Check sheet for the modelled part. Datum: model origin and axes. Units: mm. Face numbers are marked on the shaded views. A direction names the side the tool comes from. Coordinates: 2 decimals unless noted, no trailing zeros. Loops run counter-clockwise (first coordinate to the right, second up) from the corner with the lowest first, then second, coordinate; pieces in that order, holes last. Notation, with made-up numbers: (29, 20) -> (52, 20) arc R19 ccw to (52, 31) -> close; hole circle Ø6 at (83, 2.25). An arc over 180 degrees is marked (long way). Use one line per item in the form item = value.
from build123d import *

# Parameters (mm, degrees)
F3_W     = 10.7
F3_H     = 4
F4_DEPTH = 4
F5_R     = 1.99999


# Not quite as in the source:
# - a fillet or chamfer is up to 0.001 mm smaller than in the source, because OpenCascade refuses the exact size


with BuildPart() as f1:
    # F0 (on Front) → F1 (revolve)
    with BuildSketch(Plane.XZ):
        Polygon((0, 8), (0, 0), (215, 0), (215, 5), (203.5, 5), (203.5, 6), (187.5, 6), (187.5, 7.5), (172.5, 7.5), (172.5, 10.75), (168, 10.75), (168, 5.675), (161, 5.675), (161, 8), align=None)
    revolve(axis=Axis((-30.1147408886, 0, 0), (-1, 0, 0)))

    # F3 (on offset) → F4 (cut)
    with BuildSketch(Plane.XY.offset(7.5)):
        with Locations((196.15, 0)):
            Rectangle(F3_W, F3_H)
    extrude(amount=-F4_DEPTH, mode=Mode.SUBTRACT)

    # F5 (radius 2 in the source; OpenCascade refuses exactly that, so slightly less here)
    f5_edges = [f1.edges().sort_by_distance(p)[0] for p in [
        (190.8, 2, 4.578427),
        (201.5, 2, 4.578427),
        (201.5, -2, 4.578427),
        (190.8, -2, 4.578427),
    ]]
    fillet(f5_edges, radius=F5_R)


solid = f1.part
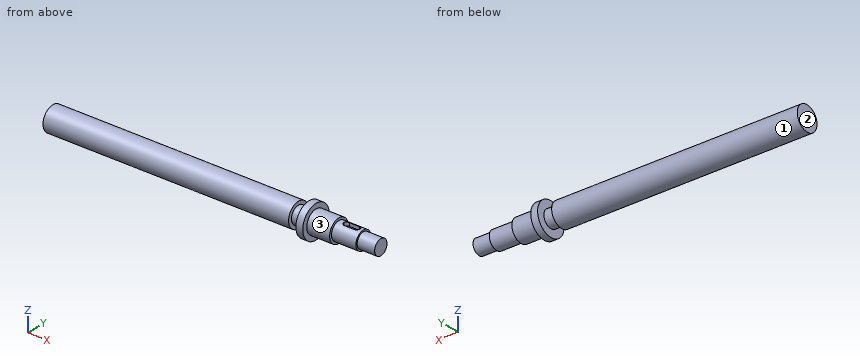
(1) Section check A-A, the plane z = 0. Record the boundary of the cut face in (x, y) (3 decimals), plus the area to 3 significant figures.
Established:
outline = (0, -8) -> (161, -8) -> (161, -5.675) -> (168, -5.675) -> (168, -10.75) -> (172.5, -10.75) -> (172.5, -7.5) -> (187.5, -7.5) -> (187.5, -6) -> (203.5, -6) -> (203.5, -5) -> (215, -5) -> (215, 5) -> (203.5, 5) -> (203.5, 6) -> (187.5, 6) -> (187.5, 7.5) -> (172.5, 7.5) -> (172.5, 10.75) -> (168, 10.75) -> (168, 5.675) -> (161, 5.675) -> (161, 8) -> (0, 8) -> close
area = 3,280 mm²
(2) Scan lines: line 1 along X through (y, z) = (-3.75, -5.75); line 2 along X through (y, z) = (3.25, 7.5); line 3 along Y through (x, z) = (180.5, 0). Record each from-to range of solid material in increasing order.
Established:
line_1 = 0 to 161, 168 to 187.5
line_2 = 168 to 172.5
line_3 = -7.5 to 7.5
(3) Tool access check on the marked faces 1, 2 and 3. Record the directions out of +Z, -Z, +X, -X, +Y, -Y that give a thin tool (end or side, any length) a straight path to the whole face; none if there is none.
Established:
face_1 = -X
face_2 = +Z, -Z, -X, +Y, -Y
face_3 = +X
(4) Go/stop test with flat-tipped pins: P1, Ø4, axis at x = 122, z = -5.5, coming from the -Y side; P2, Ø1.5, axis at x = 99.5, z = -7, coming from the -Y side; P3, Ø3, axis at x = 31.5, z = 3.5, coming from the -Y side. Record where each tip stops, or that it passes through.
Established:
P1 = -7.19
P2 = -4.99
P3 = -7.75
(5) Section check B-B, the plane x = 149. Record the boundary of the cut face in (y, z).
Established:
outline = circle Ø16 at (0, 0)
